from build123d import *

# Parameters (mm, degrees)
PAD_DEPTH    = 32
SKETCH001_W  = 15
SKETCH001_H  = 3
PAD001_DEPTH = 26
SKETCH002_W  = 19
SKETCH002_H  = 3
PAD002_DEPTH = 35
SKETCH003_W  = 15
SKETCH003_H  = 3
PAD003_DEPTH = 26
SKETCH004_W  = 19
SKETCH004_H  = 3
PAD004_DEPTH = 35
SKETCH006_W  = 15
SKETCH006_H  = 3
POCKET_DEPTH = 100


with BuildPart() as part:
    # Sketch → Pad (new body)
    with BuildSketch(Plane.XZ):
        Polygon((0, 0), (0, 33), (13, 33), (13, 0), (10, 0), (10, 30), (3, 30), (3, 0), align=None)
    extrude(amount=PAD_DEPTH)

    # Sketch001 (on Face1 of Pad) → Pad001 (join)
    with BuildSketch(Plane(origin=(0, 0, 0), x_dir=(0, 0, -1), z_dir=(-1, 0, 0))):
        with Locations((-25.5, 1.5)):
            Rectangle(SKETCH001_W, SKETCH001_H)
    extrude(amount=PAD001_DEPTH)

    # Sketch002 (on Face3 of Pad001) → Pad002 (join)
    with BuildSketch(Plane(origin=(0, 0, 18), x_dir=(1, 0, 0), z_dir=(0, 0, -1))):
        with Locations((-16.5, 1.5)):
            Rectangle(SKETCH002_W, SKETCH002_H)
    extrude(amount=PAD002_DEPTH)

    # Sketch003 (on Face1 of Pad002) → Pad003 (join)
    with BuildSketch(Plane(origin=(0, 0, 0), x_dir=(0, 0, -1), z_dir=(-1, 0, 0))):
        with Locations((-25.5, 30.5)):
            Rectangle(SKETCH003_W, SKETCH003_H)
    extrude(amount=PAD003_DEPTH)

    # Sketch004 (on Face7 of Pad003) → Pad004 (join)
    with BuildSketch(Plane(origin=(0, 0, 18), x_dir=(1, 0, 0), z_dir=(0, 0, -1))):
        with Locations((-16.5, 30.5)):
            Rectangle(SKETCH004_W, SKETCH004_H)
    extrude(amount=PAD004_DEPTH)

    # Sketch006 (on Face30 of Pad004) → Pocket (cut)
    with BuildSketch(Plane.XZ.offset(32)):
        with Locations((-16.5, -13.5)):
            Rectangle(SKETCH006_W, SKETCH006_H)
        with Locations((-16.5, -8.5)):
            Rectangle(SKETCH006_W, SKETCH006_H)
        with Locations((-16.5, -3.5)):
            Rectangle(SKETCH006_W, SKETCH006_H)
        with Locations((-16.5, 1.5)):
            Rectangle(SKETCH006_W, SKETCH006_H)
        with Locations((-16.5, 6.5)):
            Rectangle(SKETCH006_W, SKETCH006_H)
        with Locations((-16.5, 11.5)):
            Rectangle(SKETCH006_W, SKETCH006_H)
        with Locations((-16.5, 16.5)):
            Rectangle(SKETCH006_W, SKETCH006_H)
        with Locations((-16.5, 21.5)):
            Rectangle(SKETCH006_W, SKETCH006_H)
        with Locations((-16.5, 26.5)):
            Rectangle(SKETCH006_W, SKETCH006_H)
    extrude(amount=-POCKET_DEPTH, mode=Mode.SUBTRACT)


solid = part.part
Can you work these out from the model? Positions are in its coordinate system, mm. A direction names the side the tool comes from. Give positions to 0.01 mm unless a question says otherwise; leave off trailing zeros. Order: outer loops, then holes, each group sorted by start corner. A loop starts at its lowest first (then second) coordinate and runs counter-clockwise, first axis right, second up. Notation, with made-up numbers: M 1.25,44.25 L 32.25,44.25 A19 cw 32.25,51.25 Z; hole C -5.5,0 d7. An arc over 180 degrees is marked long. One line per item, written item: value.
Item 1: If we section it at A-A on z = -9: Write out the boundary of the cut face in (x, y).
Verdict:
outline: M -26,-32 L -24,-32 L -24,-29 L -26,-29 Z; M -26,-3 L -24,-3 L -24,0 L -26,0 Z; M -9,-32 L -7,-32 L -7,-29 L -9,-29 Z; M -9,-3 L -7,-3 L -7,0 L -9,0 Z
Item 2: Please list where these lines run through material, in increasing order: line 1 (X direction, y = -1.5, z = 16); line 2 (X direction, y = -28, z = 18); line 3 (X direction, y = -30, z = 29.5).
Verdict:
line 1: -26 to -24, -9 to -7, 0 to 3, 10 to 13
line 2: 0 to 3, 10 to 13
line 3: -26 to 3, 10 to 13
Item 3: If we mould it in two halves opening along Z, with no side actions, what happens to faces 1 (the face through (-24, -2, -9)), 2 (the face through (2, -16, 33)), 3 (the face through (-13, -29, 14)), 4 (the face through (-17, -2, 28))? For each: pulls with the +Z half, pulls with the -Z half, needs draft (parallel to the pull), parting line crosses it, or undercut.
Verdict:
face 1: undercut
face 2: pulls with the +Z half
face 3: needs draft
face 4: undercut
Item 4: If we section it at B-B on z = 6: Write out the boundary of the cut face in (x, y), and give its area (3 significant figures).
Verdict:
outline: M -26,-32 L -24,-32 L -24,-29 L -26,-29 Z; M -26,-3 L -24,-3 L -24,0 L -26,0 Z; M -9,-32 L -7,-32 L -7,-29 L -9,-29 Z; M -9,-3 L -7,-3 L -7,0 L -9,0 Z; M 0,-32 L 3,-32 L 3,0 L 0,0 Z; M 10,-32 L 13,-32 L 13,0 L 10,0 Z
area: 216 mm2
Item 5: For faces 5 (the face through (12, -16, 0)), 6 (the face through (-17, -31, -17)), 7 (the face through (-17, -31, 10)), which set-ups out of +Z, -Z, +X, -X, +Y, -Y let a thin tool reach every point of the face, with its end or its side?
Verdict:
face 5: -Z, +X, +Y, -Y
face 6: -Z, +X, -X, +Y, -Y
face 7: +Y, -Y
Item 6: If we section it at D-D on x = -23: State how many separate pieces and enclosed holes the cut face has, and give its area (3 significant figures).
Verdict:
separate pieces: 20
enclosed holes: 0
area: 138 mm2
Item 7: For pin 1 (9.5 mm diameter, centred on y = -18.5, z = 22.5, fed in from -X); pin 2 (2.5 mm diameter, centred on y = -2, z = -8, fed in from +X); pin 3 (3.5 mm diameter, centred on x = 1, y = -10, fed in from -Z); pin 4 (3 mm diameter, centred on x = -2.5, y = -23, fed in from +Z), each with a flat end and sliding along its axis, tell me the tip position at first contact or that it passes through.
Verdict:
pin 1: x = 0
pin 2: x = -7
pin 3: z = 0
pin 4: through
Item 8: If we section it at C-C on y = -24: Write out the boundary of the cut face in (x, z), and give its area (3 significant figures).
Verdict:
outline: M 0,0 L 3,0 L 3,30 L 10,30 L 10,0 L 13,0 L 13,33 L 0,33 Z
area: 219 mm2
